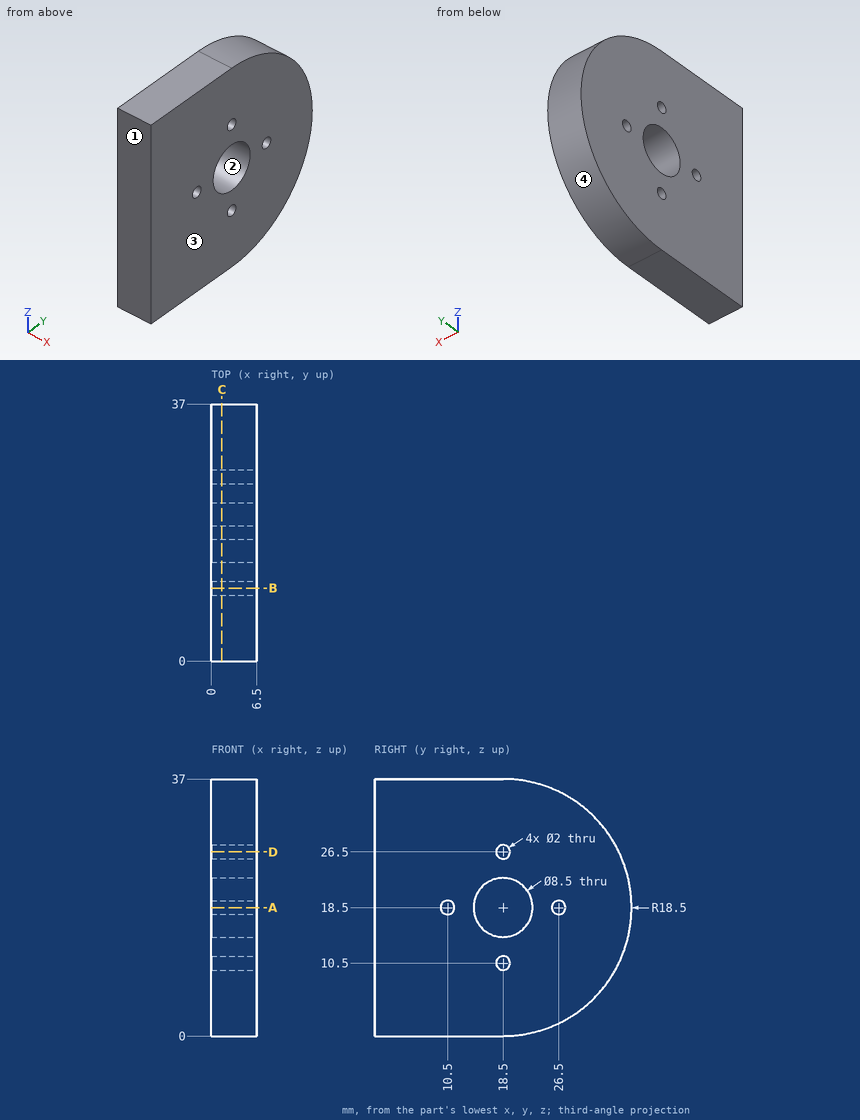
Geometry check sheet. Reference: drawing and pictorial views, mm from the part's lowest x, y, z. Give positions to 0.01 mm unless a question says otherwise; leave off trailing zeros. Order: outer loops, then holes, each group sorted by start corner. A loop starts at its lowest first (then second) coordinate and runs counter-clockwise, first axis right, second up. Notation, with made-up numbers: M 1.25,-15 L 30.25,-15 A20 cw 30.25,23 Z; hole C 47,25.25 d9. An arc over 180 degrees is marked long. Answer in a Markdown table with one row per item. Add a question column.
Item 1: Scan lines: probe 1 along Z at (x, y) = (4.25, 18.5); probe 2 along Z at (x, y) = (1.75, 10.5); probe 3 along Y at (x, z) = (5.75, 21.5). Record each from-to range of solid material in increasing order. Write a range as from..to.
Item 2: Section check A-A, the plane z = 18.5. Enter the section's corners in (x, y), and give its area (3 significant figures).
Item 3: Gauge pin test, flat ends, axial feed: pin 1 (3 mm diameter, centred on x = 5.5, z = 13.5, fed in from +Y); pin 2 (1.5 mm diameter, centred on x = 1, z = 25.5, fed in from +Y). Record the tip position at first contact, or that the pin passes through.
Item 4: Section check D-D, the plane z = 26.5. Enter the section's corners in (x, y).
Item 5: Section check C-C, the plane x = 1.5. Enter the section's corners in (y, z).
Item 6: Section check B-B, the plane y = 10.5. Enter the section's corners in (x, z), and give its area (4 significant figures).
Item 7: Mould release check, pull along Y, two halves, no side actions. Record for the marked faces 1, 2, 3 and 4: released by +Y, released by -Y, zero draft, split by the parting line, or undercut.
Filled sheet:
| question | item | result |
|---|---|---|
| 1 | probe 1 | z = 0..9.5, 11.5..14.25, 22.75..25.5, 27.5..37 |
| 1 | probe 2 | z = 0..17.5, 19.5..37 |
| 1 | probe 3 | y = 0..15.49, 21.51..36.76 |
| 2 | outline | M 0,0 L 6.5,0 L 6.5,9.5 L 0,9.5 Z; M 0,11.5 L 6.5,11.5 L 6.5,14.25 L 0,14.25 Z; M 0,22.75 L 6.5,22.75 L 6.5,25.5 L 0,25.5 Z; M 0,27.5 L 6.5,27.5 L 6.5,37 L 0,37 Z |
| 2 | area | 159 mm^2 |
| 3 | pin 1 | stops at y = 36.67 |
| 3 | pin 2 | stops at y = 35.91 |
| 4 | outline | M 0,0 L 6.5,0 L 6.5,17.5 L 0,17.5 Z; M 0,19.5 L 6.5,19.5 L 6.5,35.18 L 0,35.18 Z |
| 5 | outline | M 0,0 L 18.5,0 A18.5 ccw 18.5,37 L 0,37 Z; hole C 10.5,18.5 d2; hole C 18.5,18.5 d8.5; hole C 18.5,10.5 d2; hole C 18.5,26.5 d2; hole C 26.5,18.5 d2 |
| 6 | outline | M 0,0 L 6.5,0 L 6.5,17.5 L 0,17.5 Z; M 0,19.5 L 6.5,19.5 L 6.5,37 L 0,37 Z |
| 6 | area | 227.5 mm^2 |
| 7 | face 1 | released by -Y |
| 7 | face 2 | undercut |
| 7 | face 3 | zero draft |
| 7 | face 4 | released by +Y |
